Input: part model. Units: mm. Frame: model coordinates. Coordinates: 2 decimals unless noted, no trailing zeros. Write each loop counter-clockwise with the first axis right and the second up, starting at its lowest first coordinate (ties: lowest second). Pieces come first, ordered by that corner, then holes. Notation, with made-up numbers: M 13.5,81 L 24.5,81 A13 cw 24.5,91 Z; hole C 44,79 d1. An arc over 180 degrees is marked long. Write each question's results on one line, items separated by ' | '. Start each with the question number.
1. Section query B-B, the plane y = 0.75. Output: boundary loops of the cut face in (x, z).
2. Pull-direction query (Y, two-part tool) for faces 1 (the flat face through (-1, 1.25, 0)), 2 (the flat face through (1, -1.25, 0)), 3 (the flat face through (0, 0, 0.75)); classes: +Y half, -Y half, draft (parallel to the pull), parting line (faces both ways), or undercut.
3. Section query D-D, the plane x = 0.8. Output: boundary loops of the cut face in (y, z), and give its area (3 significant figures).
4. First-contact query: pin 1 (0.5 mm diameter, centred on x = -1, z = 2, fed in from -Y); pin 2 (0.7 mm diameter, centred on y = 0, z = -2.5, fed in from +X); pin 3 (1.5 mm diameter, centred on x = -1.5, y = 0.5, fed in from -Z); pin 4 (0.7 mm diameter, centred on x = -1.5, z = 2, fed in from +Y). Flat tips, straight axial feed; report the tip coordinate or a pass-through.
5. Ray query, probe 1 along X at (y, z) = (0.05, -5.25); probe 2 along Z at (x, y) = (1.6, 0.45); probe 3 along Z at (x, y) = (1.1, 1.05). Return the intervals inside material, ascending.
6. Section query A-A, the plane z = -3.5. Output: boundary loops of the cut face in (x, y), and give its area (3 significant figures).
7. Section query C-C, the plane z = 0.5. Output: boundary loops of the cut face in (x, y), and give its area (3 significant figures).
```python
from build123d import *
from OCP.BRepFilletAPI import BRepFilletAPI_MakeChamfer

# Parameters (mm, degrees)
EXTRUDE_1_DEPTH     = 1.25
SKETCH_2_W          = 0.5
SKETCH_2_H          = 1.3
CUT_EXTRUDE_1_DEPTH = 6.378791686
SKETCH_3_W          = 0.64
SKETCH_3_H          = 0.64
EXTRUDE_2_DEPTH     = 6
EXTRUDE_START       = -2
SKETCH_3_2_W        = 0.64
SKETCH_3_2_H        = 0.64
EXTRUDE_3_DEPTH     = 3
CHAMFER_1_SIZE      = 0.6
CHAMFER_1_SIZE2     = 0.105796188


with BuildPart() as part:
    # 草图1 → 凸台-拉伸1 (new, symmetric)
    with BuildSketch(Plane.XY):
        Polygon((-1.92, 1.25), (-2.54, 0.65), (-2.54, -0.65), (-1.92, -1.25), (-0.62, -1.25), (-0.04, -0.65), (0.04, -0.65), (0.62, -1.25), (1.92, -1.25), (2.54, -0.65), (2.54, 0.65), (1.92, 1.25), (0.62, 1.25), (0.04, 0.65), (-0.04, 0.65), (-0.62, 1.25), align=None)
    extrude(amount=EXTRUDE_1_DEPTH, both=True)

    # 草图2 → 切除-拉伸1 (cut, through all)
    with BuildSketch(Plane.ZY.offset(2.54)):
        with Locations((1, 0)):
            Rectangle(SKETCH_2_W, SKETCH_2_H)
    extrude(amount=-CUT_EXTRUDE_1_DEPTH, mode=Mode.SUBTRACT)

    # 草图3 → 凸台-拉伸2 (add)
    with BuildSketch(Plane(origin=(0, 0, -1.25), x_dir=(-1, 0, 0), z_dir=(0, 0, -1))):
        with Locations((-1.27, 0)):
            Rectangle(SKETCH_3_W, SKETCH_3_H)
        with Locations((1.27, 0)):
            Rectangle(SKETCH_3_W, SKETCH_3_H)
    extrude(amount=EXTRUDE_2_DEPTH)

    # 草图3<2> → 凸台-拉伸3 (add)
    with BuildSketch(Plane(origin=(0, 0, -1.25), x_dir=(-1, 0, 0), z_dir=(0, 0, -1)).offset(EXTRUDE_START)):
        with Locations((-1.27, 0)):
            Rectangle(SKETCH_3_2_W, SKETCH_3_2_H)
        with Locations((1.27, 0)):
            Rectangle(SKETCH_3_2_W, SKETCH_3_2_H)
    extrude(amount=-EXTRUDE_3_DEPTH)

    # 倒角1: one chamfer whose edges measure the first distance from different faces: ONE call of the kernel's chamfer builder (chamfer() names one face for all edges)
    chamfer_1_edges_1 = [part.edges().sort_by_distance(p)[0] for p in [
        (-1.59, 0, 3.75),
    ]]
    chamfer_1_side_1 = [part.faces().sort_by_distance(p)[0] for p in [
        (-1.59, 0, 2.25),
    ]]
    chamfer_1_edges_2 = [part.edges().sort_by_distance(p)[0] for p in [
        (-1.27, -0.32, 3.75),
    ]]
    chamfer_1_side_2 = [part.faces().sort_by_distance(p)[0] for p in [
        (-1.27, -0.32, 2.25),
    ]]
    chamfer_1_edges_3 = [part.edges().sort_by_distance(p)[0] for p in [
        (-0.95, 0, 3.75),
    ]]
    chamfer_1_side_3 = [part.faces().sort_by_distance(p)[0] for p in [
        (-0.95, 0, 2.25),
    ]]
    chamfer_1_edges_4 = [part.edges().sort_by_distance(p)[0] for p in [
        (-1.27, 0.32, 3.75),
    ]]
    chamfer_1_side_4 = [part.faces().sort_by_distance(p)[0] for p in [
        (-1.27, 0.32, 2.25),
    ]]
    chamfer_1_edges_5 = [part.edges().sort_by_distance(p)[0] for p in [
        (1.59, 0, -7.25),
    ]]
    chamfer_1_side_5 = [part.faces().sort_by_distance(p)[0] for p in [
        (1.59, 0, -4.25),
    ]]
    chamfer_1_edges_6 = [part.edges().sort_by_distance(p)[0] for p in [
        (1.27, -0.32, -7.25),
    ]]
    chamfer_1_side_6 = [part.faces().sort_by_distance(p)[0] for p in [
        (1.27, -0.32, -4.25),
    ]]
    chamfer_1_edges_7 = [part.edges().sort_by_distance(p)[0] for p in [
        (0.95, 0, -7.25),
    ]]
    chamfer_1_side_7 = [part.faces().sort_by_distance(p)[0] for p in [
        (0.95, 0, -4.25),
    ]]
    chamfer_1_edges_8 = [part.edges().sort_by_distance(p)[0] for p in [
        (1.27, 0.32, -7.25),
    ]]
    chamfer_1_side_8 = [part.faces().sort_by_distance(p)[0] for p in [
        (1.27, 0.32, -4.25),
    ]]
    chamfer_1_edges_9 = [part.edges().sort_by_distance(p)[0] for p in [
        (-1.59, 0, -7.25),
    ]]
    chamfer_1_side_9 = [part.faces().sort_by_distance(p)[0] for p in [
        (-1.59, 0, -4.25),
    ]]
    chamfer_1_edges_10 = [part.edges().sort_by_distance(p)[0] for p in [
        (-1.27, 0.32, -7.25),
    ]]
    chamfer_1_side_10 = [part.faces().sort_by_distance(p)[0] for p in [
        (-1.27, 0.32, -4.25),
    ]]
    chamfer_1_edges_11 = [part.edges().sort_by_distance(p)[0] for p in [
        (-0.95, 0, -7.25),
    ]]
    chamfer_1_side_11 = [part.faces().sort_by_distance(p)[0] for p in [
        (-0.95, 0, -4.25),
    ]]
    chamfer_1_edges_12 = [part.edges().sort_by_distance(p)[0] for p in [
        (-1.27, -0.32, -7.25),
    ]]
    chamfer_1_side_12 = [part.faces().sort_by_distance(p)[0] for p in [
        (-1.27, -0.32, -4.25),
    ]]
    chamfer_1_edges_13 = [part.edges().sort_by_distance(p)[0] for p in [
        (1.59, 0, 3.75),
    ]]
    chamfer_1_side_13 = [part.faces().sort_by_distance(p)[0] for p in [
        (1.59, 0, 2.25),
    ]]
    chamfer_1_edges_14 = [part.edges().sort_by_distance(p)[0] for p in [
        (1.27, 0.32, 3.75),
    ]]
    chamfer_1_side_14 = [part.faces().sort_by_distance(p)[0] for p in [
        (1.27, 0.32, 2.25),
    ]]
    chamfer_1_edges_15 = [part.edges().sort_by_distance(p)[0] for p in [
        (0.95, 0, 3.75),
    ]]
    chamfer_1_side_15 = [part.faces().sort_by_distance(p)[0] for p in [
        (0.95, 0, 2.25),
    ]]
    chamfer_1_edges_16 = [part.edges().sort_by_distance(p)[0] for p in [
        (1.27, -0.32, 3.75),
    ]]
    chamfer_1_side_16 = [part.faces().sort_by_distance(p)[0] for p in [
        (1.27, -0.32, 2.25),
    ]]
    chamfer_1 = BRepFilletAPI_MakeChamfer(part.part.solid().wrapped)
    for e in chamfer_1_edges_1:
        chamfer_1.Add(CHAMFER_1_SIZE, CHAMFER_1_SIZE2, e.wrapped, chamfer_1_side_1[0].wrapped)  # the first distance lies on this face
    for e in chamfer_1_edges_2:
        chamfer_1.Add(CHAMFER_1_SIZE, CHAMFER_1_SIZE2, e.wrapped, chamfer_1_side_2[0].wrapped)  # the first distance lies on this face
    for e in chamfer_1_edges_3:
        chamfer_1.Add(CHAMFER_1_SIZE, CHAMFER_1_SIZE2, e.wrapped, chamfer_1_side_3[0].wrapped)  # the first distance lies on this face
    for e in chamfer_1_edges_4:
        chamfer_1.Add(CHAMFER_1_SIZE, CHAMFER_1_SIZE2, e.wrapped, chamfer_1_side_4[0].wrapped)  # the first distance lies on this face
    for e in chamfer_1_edges_5:
        chamfer_1.Add(CHAMFER_1_SIZE, CHAMFER_1_SIZE2, e.wrapped, chamfer_1_side_5[0].wrapped)  # the first distance lies on this face
    for e in chamfer_1_edges_6:
        chamfer_1.Add(CHAMFER_1_SIZE, CHAMFER_1_SIZE2, e.wrapped, chamfer_1_side_6[0].wrapped)  # the first distance lies on this face
    for e in chamfer_1_edges_7:
        chamfer_1.Add(CHAMFER_1_SIZE, CHAMFER_1_SIZE2, e.wrapped, chamfer_1_side_7[0].wrapped)  # the first distance lies on this face
    for e in chamfer_1_edges_8:
        chamfer_1.Add(CHAMFER_1_SIZE, CHAMFER_1_SIZE2, e.wrapped, chamfer_1_side_8[0].wrapped)  # the first distance lies on this face
    for e in chamfer_1_edges_9:
        chamfer_1.Add(CHAMFER_1_SIZE, CHAMFER_1_SIZE2, e.wrapped, chamfer_1_side_9[0].wrapped)  # the first distance lies on this face
    for e in chamfer_1_edges_10:
        chamfer_1.Add(CHAMFER_1_SIZE, CHAMFER_1_SIZE2, e.wrapped, chamfer_1_side_10[0].wrapped)  # the first distance lies on this face
    for e in chamfer_1_edges_11:
        chamfer_1.Add(CHAMFER_1_SIZE, CHAMFER_1_SIZE2, e.wrapped, chamfer_1_side_11[0].wrapped)  # the first distance lies on this face
    for e in chamfer_1_edges_12:
        chamfer_1.Add(CHAMFER_1_SIZE, CHAMFER_1_SIZE2, e.wrapped, chamfer_1_side_12[0].wrapped)  # the first distance lies on this face
    for e in chamfer_1_edges_13:
        chamfer_1.Add(CHAMFER_1_SIZE, CHAMFER_1_SIZE2, e.wrapped, chamfer_1_side_13[0].wrapped)  # the first distance lies on this face
    for e in chamfer_1_edges_14:
        chamfer_1.Add(CHAMFER_1_SIZE, CHAMFER_1_SIZE2, e.wrapped, chamfer_1_side_14[0].wrapped)  # the first distance lies on this face
    for e in chamfer_1_edges_15:
        chamfer_1.Add(CHAMFER_1_SIZE, CHAMFER_1_SIZE2, e.wrapped, chamfer_1_side_15[0].wrapped)  # the first distance lies on this face
    for e in chamfer_1_edges_16:
        chamfer_1.Add(CHAMFER_1_SIZE, CHAMFER_1_SIZE2, e.wrapped, chamfer_1_side_16[0].wrapped)  # the first distance lies on this face
    add(Compound.cast(chamfer_1.Shape()), mode=Mode.REPLACE)


solid = part.part
```
Answer:
1) outline: M -2.44,-1.25 L -0.14,-1.25 L -0.14,1.25 L -2.44,1.25 Z; M 0.14,-1.25 L 2.44,-1.25 L 2.44,1.25 L 0.14,1.25 Z
2) face 1: +Y half | face 2: -Y half | face 3: undercut
3) outline: M -1.25,-1.25 L 1.25,-1.25 L 1.25,1.25 L 0.65,1.25 L 0.65,0.75 L -0.65,0.75 L -0.65,1.25 L -1.25,1.25 Z | area: 5.60 mm^2
4) pin 1: y = -0.32 | pin 2: x = 1.59 | pin 3: z = -7.25 | pin 4: y = 0.32
5) probe 1: -1.59 to -0.95, 0.95 to 1.59 | probe 2: -1.25 to 0.75 | probe 3: -1.25 to 1.25
6) outline: M -1.59,-0.32 L -0.95,-0.32 L -0.95,0.32 L -1.59,0.32 Z; M 0.95,-0.32 L 1.59,-0.32 L 1.59,0.32 L 0.95,0.32 Z | area: 0.819 mm^2
7) outline: M -2.54,-0.65 L -1.92,-1.25 L -0.62,-1.25 L -0.04,-0.65 L 0.04,-0.65 L 0.62,-1.25 L 1.92,-1.25 L 2.54,-0.65 L 2.54,0.65 L 1.92,1.25 L 0.62,1.25 L 0.04,0.65 L -0.04,0.65 L -0.62,1.25 L -1.92,1.25 L -2.54,0.65 Z | area: 11.2 mm^2
